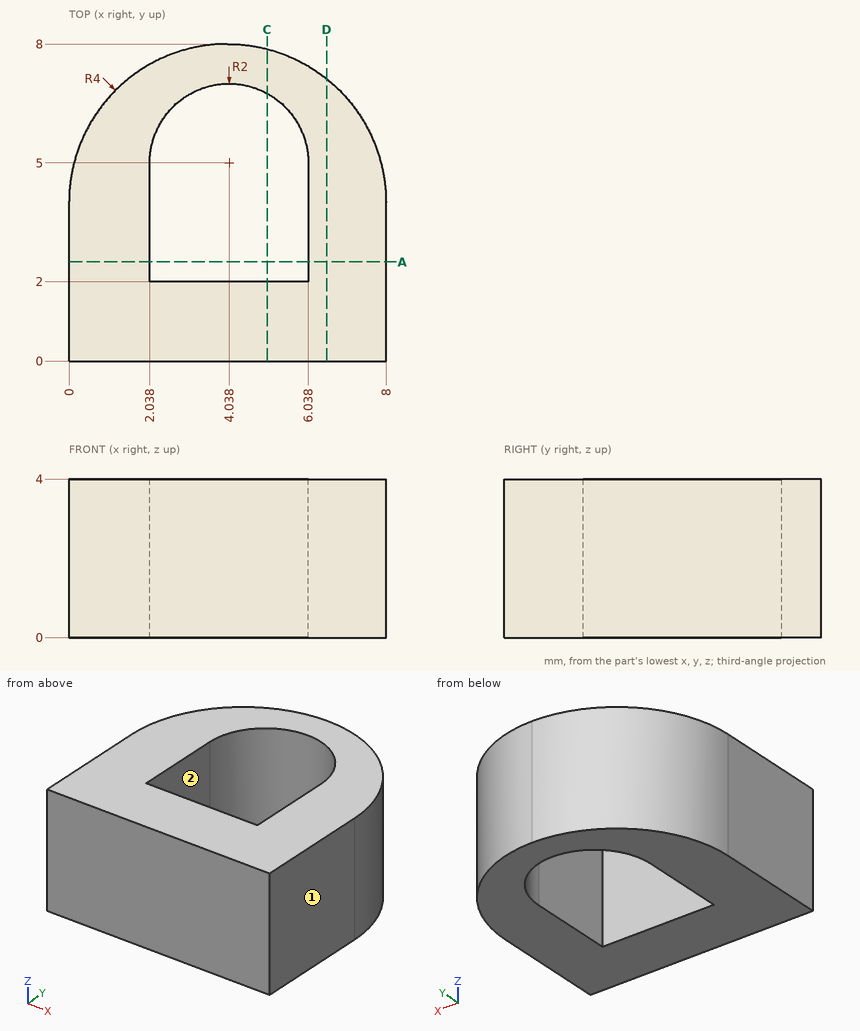
For this review, use the dimensioned drawing (mm, ordinates from the lowest corner) and the shaded views. A direction names the side the tool comes from. Round coordinates to 2 decimals unless told otherwise and drop trailing zeros. Order: outer loops, then holes, each group sorted by start corner. A loop starts at its lowest first (then second) coordinate and runs counter-clockwise, first axis right, second up. Notation, with made-up numbers: M -7.75,72.25 L 41.25,72.25 A13 ccw 41.25,94.25 Z; hole C -31.75,-17.5 d8. An arc over 180 degrees is marked long. Use a Markdown table: item, result.
1) Tool access review of the marked faces 1 and 2: name each direction out of +Z, -Z, +X, -X, +Y, -Y from which nothing blocks a thin tool from reaching the whole face with its end or side.
Report:
| item | result |
|---|---|
| face 1 | +Z, -Z, +X, +Y, -Y |
| face 2 | +Z, -Z |
2) Consider section C-C (x = 5). Write out the cut boundary in (y, z), then the cut area to 3 significant figures.
Report:
| item | result |
|---|---|
| outline | M 0,0 L 2,0 L 2,4 L 0,4 Z; M 6.75,0 L 7.87,0 L 7.87,4 L 6.75,4 Z |
| area | 12.5 mm^2 |
3) Consider section A-A (y = 2.5). Write out the cut boundary in (x, z).
Report:
| item | result |
|---|---|
| outline | M 0,0 L 2.04,0 L 2.04,4 L 0,4 Z; M 6.04,0 L 8,0 L 8,4 L 6.04,4 Z |
4) Consider section D-D (x = 6.5). Write out the cut boundary in (y, z).
Report:
| item | result |
|---|---|
| outline | M 0,0 L 7.12,0 L 7.12,4 L 0,4 Z |
5) Wall thickness on line 1 along X through (y, z) = (3.75, 1.8); line 2 along X through (y, z) = (5.75, 1.1); line 3 along Y through (x, z) = (4.5, 1.65): over which ranges is each line inside the solid? List them lowest first. Write a range as [from, to].
Report:
| item | result |
|---|---|
| line 1 | [0, 2.04], [6.04, 8] |
| line 2 | [0.4, 2.18], [5.89, 7.6] |
| line 3 | [0, 2], [6.95, 7.97] |
